```python
from build123d import *

# Parameters (mm, degrees)
F1_DEPTH      = 19.05
F2_W          = 6.35
F2_H          = 7.62
F3_DEPTH      = 25.401
F3_DEPTH_BACK = 25.4


with BuildPart() as f1:
    # F0 (on Top) → F1 (new body)
    with BuildSketch(Plane.XY):
        Polygon((25.4, 0), (0, 0), (-25.4, 0), (-10.7353031626, -25.4), (-25.4, -50.8), (0, -50.8), (25.4, -50.8), (10.7353031626, -25.4), align=None)
    extrude(amount=F1_DEPTH)

    # F2 (on Right) → F3 (cut, two sides)
    with BuildSketch(Plane.YZ) as f3_sk:
        with Locations((-3.175, 3.81)):
            Rectangle(F2_W, F2_H)
        with Locations((-47.625, 3.81)):
            Rectangle(F2_W, F2_H)
    extrude(amount=-F3_DEPTH, mode=Mode.SUBTRACT)
    extrude(f3_sk.sketch, amount=F3_DEPTH_BACK, mode=Mode.SUBTRACT)


solid = f1.part
```
The model under review builds one solid part; all positions refer to its coordinate system, in mm. A direction names the side the tool comes from. Round coordinates to 2 decimals unless told otherwise and drop trailing zeros. Loops run counter-clockwise (first coordinate to the right, second up) from the corner with the lowest first, then second, coordinate; pieces in that order, holes last. Notation, with made-up numbers: (48, -4) - (61, -4) arc R32 cw to (61, 31) - close; hole circle Ø4 at (-35.75, 66.25). An arc over 180 degrees is marked (long way). Use a Markdown table: item, result. Add a question column.
Q1. Add section D-D (y = -17). State the section outline as (x, z) points.
Q2. Machinability: for faces 5 (the face through (17.965, -12.878, 9.392)), 6 (the face through (0, -48, 7.62)), 7 (the face through (-17.965, -37.922, 9.392)), 8 (the face through (0, -6.35, 4)), which of the approach directions +Z, -Z, +X, -X, +Y, -Y give a long, thin tool a straight path to every point of the face, cutting with its end or side? Answer none if there is none.
Q3. The part is to be moulded in two halves that separate along Y. For faces 1 (the face through (0, -3, 7.62)), 2 (the face through (0, -44.45, 4)), 3 (the face through (0, 0, 13)), 4 (the face through (-18.17, -12.52, 9.39)), say which applies: pulls with the +Y half, pulls with the -Y half, needs draft (parallel to the pull), parting line crosses it, or undercut.
Q4. Add section C-C (x = -20). State the section outline as (y, z) points.
Q5. For probe 1 along Y at (x, z) = (1, 4.5); probe 2 along Y at (x, z) = (17.5, 4); probe 3 along Y at (x, z) = (-15.5, 16.5), list the stretches that pass through material, from the lowest coordinate up.
Q6. Add section A-A (z = 2). State the section outline as (x, y) points, plus the area to 3 significant figures.
Q7. Insertion check: pin 1 Ø6 at (x, z) = (-6.5, 3.5) entering from -Y; pin 2 Ø5 at (y, z) = (-30.5, 8.5) entering from -X; pin 3 Ø4 at (x, y) = (-19, -13) entering from -Z; pin 4 Ø2.5 at (x, z) = (4.5, 4) entering from +Y. Each pin has a flat end and moves straight along its axis. Give the tip position at first contact, or say it passes through.
Q8. Add section B-B (x = -1). State the section outline as (y, z) points.
Worked answers:
| question | item | result |
|---|---|---|
| 1 | outline | (-15.59, 0) - (15.59, 0) - (15.59, 19.05) - (-15.59, 19.05) - close |
| 2 | face 5 | +Z, -Z, +X |
| 2 | face 6 | -Z, +X, -X, -Y |
| 2 | face 7 | +Z, -Z, -X |
| 2 | face 8 | -Z, +X, -X, +Y |
| 3 | face 1 | needs draft |
| 3 | face 2 | pulls with the -Y half |
| 3 | face 3 | pulls with the +Y half |
| 3 | face 4 | undercut |
| 4 | outline | (-50.8, 7.62) - (-44.45, 7.62) - (-44.45, 0) - (-41.45, 0) - (-41.45, 19.05) - (-50.8, 19.05) - close; (-9.35, 0) - (-6.35, 0) - (-6.35, 7.62) - (0, 7.62) - (0, 19.05) - (-9.35, 19.05) - close |
| 5 | probe 1 | -44.45 to -6.35 |
| 5 | probe 2 | -44.45 to -37.12, -13.68 to -6.35 |
| 5 | probe 3 | -50.8 to -33.65, -17.15 to 0 |
| 6 | outline | (-21.73, -44.45) - (21.73, -44.45) - (10.74, -25.4) - (21.73, -6.35) - (-21.73, -6.35) - (-10.74, -25.4) - close |
| 6 | area | 1,240 mm² |
| 7 | pin 1 | y = -44.45 |
| 7 | pin 2 | x = -15.12 |
| 7 | pin 3 | z = 0 |
| 7 | pin 4 | y = -6.35 |
| 8 | outline | (-50.8, 7.62) - (-44.45, 7.62) - (-44.45, 0) - (-6.35, 0) - (-6.35, 7.62) - (0, 7.62) - (0, 19.05) - (-50.8, 19.05) - close |
